Geometry: final body of the model. Coordinates: model frame, mm. Face numbers are marked on the shaded views. Give positions to 0.01 mm unless a question says otherwise; leave off trailing zeros. Order: outer loops, then holes, each group sorted by start corner. A loop starts at its lowest first (then second) coordinate and runs counter-clockwise, first axis right, second up. Notation, with made-up numbers: (26.5, 35) - (64.5, 35) arc R14 cw to (64.5, 52) - close; hole circle Ø6 at (-6, 59). An arc over 180 degrees is marked (long way). Put each result on its own line as item: value. Start each with the question number.
1. Ray query, line 1 along Z through (x, y) = (51, 30); line 2 along Y through (x, z) = (25, 50.75). Return the intervals inside material, ascending. Write a range as from..to.
2. Section D-D on x = -41.5. Return the cut outline in (y, z).
3. Section B-B on x = 25. Count the separate pieces of the cut face and the enclosed holes in it, plus the area to 3 significant figures.
4. First-contact query: P1, Ø3, axis at x = -0.5, z = -1.5, coming from the +Y side; P2, Ø5, axis at x = 16, z = 25, coming from the +Y side. Flat tips, straight axial feed; report the tip coordinate or a pass-through.
5. Mould query, pull axis X, two halves, no side actions, for the marked faces 1, 2, 3 and 4. Classes: pulls with the +X half, pulls with the -X half, needs draft (parallel to the pull), parting line crosses it, or undercut.
6. Section A-A on y = 64. Return the cut outline in (x, z).
from build123d import *

# Parameters (mm, degrees)
SKETCH2_W           = 105
SKETCH2_H           = 105
BOSS_EXTRUDE2_DEPTH = 110
SKETCH3_W           = 100
SKETCH3_H           = 100
CUT_EXTRUDE1_DEPTH  = 105
SKETCH4_R           = 2.5
CUT_EXTRUDE2_DEPTH  = 5
SKETCH5_R           = 2.5
CUT_EXTRUDE3_DEPTH  = 5
SKETCH6_R           = 2.5
CUT_EXTRUDE4_DEPTH  = 5
SKETCH7_R           = 2.5
CUT_EXTRUDE5_DEPTH  = 5
SKETCH8_R           = 2.5
CUT_EXTRUDE12_DEPTH = 5
SKETCH13_R          = 2.5
CUT_EXTRUDE13_DEPTH = 5
SKETCH14_R          = 2.5
CUT_EXTRUDE14_DEPTH = 5
SKETCH15_R          = 2.5
CUT_EXTRUDE15_DEPTH = 5
SKETCH16_R          = 2.5
CUT_EXTRUDE16_DEPTH = 5
SKETCH17_R          = 2.5
CUT_EXTRUDE17_DEPTH = 5
SKETCH18_R          = 2.5
CUT_EXTRUDE18_DEPTH = 5
SKETCH19_R          = 2.5
CUT_EXTRUDE19_DEPTH = 5
CUT_EXTRUDE20_START = -5
SKETCH20_R          = 2.5
CUT_EXTRUDE20_DEPTH = 5
CUT_EXTRUDE21_START = -5
SKETCH21_R          = 2.5
CUT_EXTRUDE21_DEPTH = 5
CUT_EXTRUDE22_START = -5
SKETCH22_R          = 2.5
CUT_EXTRUDE22_DEPTH = 5
CUT_EXTRUDE23_START = -5
SKETCH23_R          = 2.5
CUT_EXTRUDE23_DEPTH = 5
CUT_EXTRUDE24_START = -5
SKETCH24_R          = 2.5
CUT_EXTRUDE24_DEPTH = 5
CUT_EXTRUDE25_START = -5
SKETCH25_R          = 2.5
CUT_EXTRUDE25_DEPTH = 5
CUT_EXTRUDE26_START = -5
SKETCH26_R          = 2.5
CUT_EXTRUDE26_DEPTH = 5
CUT_EXTRUDE27_START = -5
SKETCH27_R          = 2.5
CUT_EXTRUDE27_DEPTH = 5
SKETCH28_W          = 20
SKETCH28_H          = 10
BOSS_EXTRUDE3_DEPTH = 70


with BuildPart() as part:
    # Sketch2 → Boss-Extrude2 (new body)
    with BuildSketch(Plane(origin=(0, 0, 0), x_dir=(1, 0, 0), z_dir=(0, 1, 0))):
        Rectangle(SKETCH2_W, SKETCH2_H)
    extrude(amount=BOSS_EXTRUDE2_DEPTH)

    # Sketch3 → Cut-Extrude1 (cut)
    with BuildSketch(Plane(origin=(0, 110, 0), x_dir=(1, 0, 0), z_dir=(0, 1, 0))):
        Rectangle(SKETCH3_W, SKETCH3_H)
    extrude(amount=-CUT_EXTRUDE1_DEPTH, mode=Mode.SUBTRACT)

    # Sketch4 → Cut-Extrude2 (cut)
    with BuildSketch(Plane(origin=(0, 5, 0), x_dir=(1, 0, 0), z_dir=(0, 1, 0))):
        with Locations(Location((-25, 25, 0), (0, 0, 270))):
            Circle(SKETCH4_R)
    extrude(amount=-CUT_EXTRUDE2_DEPTH, mode=Mode.SUBTRACT)

    # Sketch5 → Cut-Extrude3 (cut)
    with BuildSketch(Plane.XZ):
        with Locations(Location((25, -25, 0), (0, 0, 270))):
            Circle(SKETCH5_R)
    extrude(amount=-CUT_EXTRUDE3_DEPTH, mode=Mode.SUBTRACT)

    # Sketch6 → Cut-Extrude4 (cut)
    with BuildSketch(Plane.XZ):
        with Locations(Location((25, 25, 0), (0, 0, 270))):
            Circle(SKETCH6_R)
    extrude(amount=-CUT_EXTRUDE4_DEPTH, mode=Mode.SUBTRACT)

    # Sketch7 → Cut-Extrude5 (cut)
    with BuildSketch(Plane.XZ):
        with Locations(Location((-25, 25, 0), (0, 0, 270))):
            Circle(SKETCH7_R)
    extrude(amount=-CUT_EXTRUDE5_DEPTH, mode=Mode.SUBTRACT)

    # Sketch8 → Cut-Extrude12 (cut)
    with BuildSketch(Plane.ZY.offset(52.5)):
        with Locations((-25, 80)):
            Circle(SKETCH8_R)
    extrude(amount=-CUT_EXTRUDE12_DEPTH, mode=Mode.SUBTRACT)

    # Sketch13 → Cut-Extrude13 (cut)
    with BuildSketch(Plane.ZY.offset(52.5)):
        with Locations((-25, 30)):
            Circle(SKETCH13_R)
    extrude(amount=-CUT_EXTRUDE13_DEPTH, mode=Mode.SUBTRACT)

    # Sketch14 → Cut-Extrude14 (cut)
    with BuildSketch(Plane.ZY.offset(52.5)):
        with Locations((25, 80)):
            Circle(SKETCH14_R)
    extrude(amount=-CUT_EXTRUDE14_DEPTH, mode=Mode.SUBTRACT)

    # Sketch15 → Cut-Extrude15 (cut)
    with BuildSketch(Plane.ZY.offset(52.5)):
        with Locations((25, 30)):
            Circle(SKETCH15_R)
    extrude(amount=-CUT_EXTRUDE15_DEPTH, mode=Mode.SUBTRACT)

    # Sketch16 → Cut-Extrude16 (cut)
    with BuildSketch(Plane(origin=(0, 0, -52.5), x_dir=(-1, 0, 0), z_dir=(0, 0, -1))):
        with Locations((25, 80)):
            Circle(SKETCH16_R)
    extrude(amount=-CUT_EXTRUDE16_DEPTH, mode=Mode.SUBTRACT)

    # Sketch17 → Cut-Extrude17 (cut)
    with BuildSketch(Plane(origin=(0, 0, -52.5), x_dir=(-1, 0, 0), z_dir=(0, 0, -1))):
        with Locations((25, 30)):
            Circle(SKETCH17_R)
    extrude(amount=-CUT_EXTRUDE17_DEPTH, mode=Mode.SUBTRACT)

    # Sketch18 → Cut-Extrude18 (cut)
    with BuildSketch(Plane(origin=(0, 0, -52.5), x_dir=(-1, 0, 0), z_dir=(0, 0, -1))):
        with Locations((-25, 80)):
            Circle(SKETCH18_R)
    extrude(amount=-CUT_EXTRUDE18_DEPTH, mode=Mode.SUBTRACT)

    # Sketch19 → Cut-Extrude19 (cut)
    with BuildSketch(Plane(origin=(0, 0, -52.5), x_dir=(-1, 0, 0), z_dir=(0, 0, -1))):
        with Locations((-25, 30)):
            Circle(SKETCH19_R)
    extrude(amount=-CUT_EXTRUDE19_DEPTH, mode=Mode.SUBTRACT)

    # Sketch20 → Cut-Extrude20 (cut)
    with BuildSketch(Plane(origin=(52.5, 0, 0), x_dir=(0, 0, -1), z_dir=(1, 0, 0)).offset(CUT_EXTRUDE20_START)):
        with Locations(Location((25, 80, 0), (0, 0, 180))):
            Circle(SKETCH20_R)
    extrude(amount=CUT_EXTRUDE20_DEPTH, mode=Mode.SUBTRACT)

    # Sketch21 → Cut-Extrude21 (cut)
    with BuildSketch(Plane(origin=(52.5, 0, 0), x_dir=(0, 0, -1), z_dir=(1, 0, 0)).offset(CUT_EXTRUDE21_START)):
        with Locations(Location((-25, 80, 0), (0, 0, 180))):
            Circle(SKETCH21_R)
    extrude(amount=CUT_EXTRUDE21_DEPTH, mode=Mode.SUBTRACT)

    # Sketch22 → Cut-Extrude22 (cut)
    with BuildSketch(Plane(origin=(52.5, 0, 0), x_dir=(0, 0, -1), z_dir=(1, 0, 0)).offset(CUT_EXTRUDE22_START)):
        with Locations(Location((25, 30, 0), (0, 0, 180))):
            Circle(SKETCH22_R)
    extrude(amount=CUT_EXTRUDE22_DEPTH, mode=Mode.SUBTRACT)

    # Sketch23 → Cut-Extrude23 (cut)
    with BuildSketch(Plane(origin=(52.5, 0, 0), x_dir=(0, 0, -1), z_dir=(1, 0, 0)).offset(CUT_EXTRUDE23_START)):
        with Locations(Location((-25, 30, 0), (0, 0, 180))):
            Circle(SKETCH23_R)
    extrude(amount=CUT_EXTRUDE23_DEPTH, mode=Mode.SUBTRACT)

    # Sketch24 → Cut-Extrude24 (cut)
    with BuildSketch(Plane.XY.offset(52.5).offset(CUT_EXTRUDE24_START)):
        with Locations(Location((-25, 80, 0), (0, 0, 180))):
            Circle(SKETCH24_R)
    extrude(amount=CUT_EXTRUDE24_DEPTH, mode=Mode.SUBTRACT)

    # Sketch25 → Cut-Extrude25 (cut)
    with BuildSketch(Plane.XY.offset(52.5).offset(CUT_EXTRUDE25_START)):
        with Locations(Location((25, 80, 0), (0, 0, 180))):
            Circle(SKETCH25_R)
    extrude(amount=CUT_EXTRUDE25_DEPTH, mode=Mode.SUBTRACT)

    # Sketch26 → Cut-Extrude26 (cut)
    with BuildSketch(Plane.XY.offset(52.5).offset(CUT_EXTRUDE26_START)):
        with Locations(Location((-25, 30, 0), (0, 0, 180))):
            Circle(SKETCH26_R)
    extrude(amount=CUT_EXTRUDE26_DEPTH, mode=Mode.SUBTRACT)

    # Sketch27 → Cut-Extrude27 (cut)
    with BuildSketch(Plane.XY.offset(52.5).offset(CUT_EXTRUDE27_START)):
        with Locations(Location((25, 30, 0), (0, 0, 180))):
            Circle(SKETCH27_R)
    extrude(amount=CUT_EXTRUDE27_DEPTH, mode=Mode.SUBTRACT)

    # Sketch28 → Boss-Extrude3 (add)
    with BuildSketch(Plane(origin=(0, 5, 0), x_dir=(1, 0, 0), z_dir=(0, 1, 0))):
        Rectangle(SKETCH28_W, SKETCH28_H)
    extrude(amount=BOSS_EXTRUDE3_DEPTH)


solid = part.part
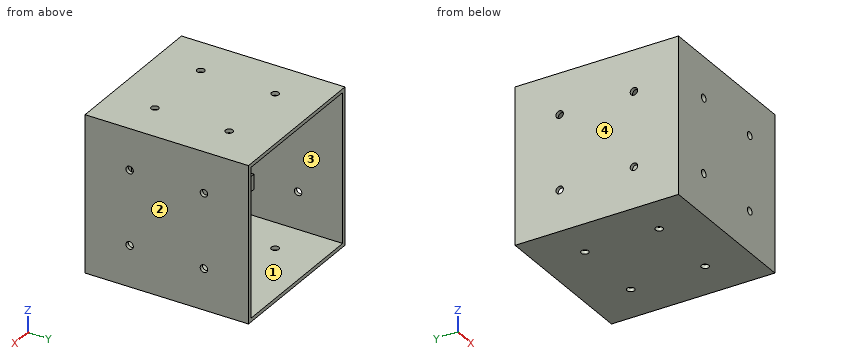
Resolved:
1. line 1: -52.5..-27.5, -22.5..22.5, 27.5..52.5
1. line 2: 0..27.5, 32.5..77.5, 82.5..110
2. outline: (0, -52.5) - (110, -52.5) - (110, -50) - (5, -50) - (5, 50) - (110, 50) - (110, 52.5) - (0, 52.5) - close
3. separate pieces: 7
3. enclosed holes: 0
3. area: 950 mm^2
4. P1: y = 75
4. P2: y = 5
5. face 1: undercut
5. face 2: pulls with the +X half
5. face 3: undercut
5. face 4: pulls with the -X half
6. outline: (-52.5, -52.5) - (52.5, -52.5) - (52.5, 52.5) - (-52.5, 52.5) - close; (-10, -5) - (10, -5) - (10, 5) - (-10, 5) - close; hole (-50, -50) - (50, -50) - (50, 50) - (-50, 50) - close
